```python
from build123d import *

# Parameters (mm, degrees)
F0_R            = 8
F1_DEPTH        = 5
F3_DEPTH        = 5
F3_COPIES_COUNT = 18
F4_R            = 2


# Not quite as in the source:
# - a pattern or mirror of a feature is missing from the dataset's text; its kind, count and spacing are read off the source's solid


with BuildPart() as f1:
    # F0 (on Top) → F1 (new body)
    with BuildSketch(Plane.XY):
        with BuildLine():
            Line((-25, -3), (-10.5830052443, -3))
            ThreePointArc((-10.5830052443, -3), (0, -11), (10.5830052443, -3))
            Line((10.5830052443, -3), (25, -3))
            Line((25, -3), (25, 3))
            Line((25, 3), (10.5830052443, 3))
            ThreePointArc((10.5830052443, 3), (0, 11), (-10.5830052443, 3))
            Line((-10.5830052443, 3), (-25, 3))
            Line((-25, 3), (-25, -3))
        make_face()
        Circle(F0_R, mode=Mode.SUBTRACT)
    extrude(amount=F1_DEPTH)

    # F2 (on Top) → F3 (join)
    with BuildSketch(Plane.XY):
        with BuildLine():
            Line((0, -7.5), (-0.2060079166, -7.9973471063))
            ThreePointArc((-0.2060079166, -7.9973471063), (0, -8), (0.2060079166, -7.9973471063))
            Line((0.2060079166, -7.9973471063), (0, -7.5))
        make_face()
    f3 = extrude(amount=F3_DEPTH)

    # F3_copies: F3 ×18 about axis
    f3_copies_axis = Axis((0, 0, 0), (0, 0, 1))
    for i in range(1, F3_COPIES_COUNT):
        add(f3.rotate(f3_copies_axis, i * 360 / F3_COPIES_COUNT))

    # F4
    f4_edges = [f1.edges().sort_by_distance(p)[0] for p in [
        (-25, 3, 2.5),
        (-25, -3, 2.5),
        (25, 3, 2.5),
        (-10.583005, 3, 2.5),
        (25, -3, 2.5),
        (10.583005, -3, 2.5),
        (-10.583005, -3, 2.5),
        (10.583005, 3, 2.5),
    ]]
    fillet(f4_edges, radius=F4_R)


solid = f1.part
```
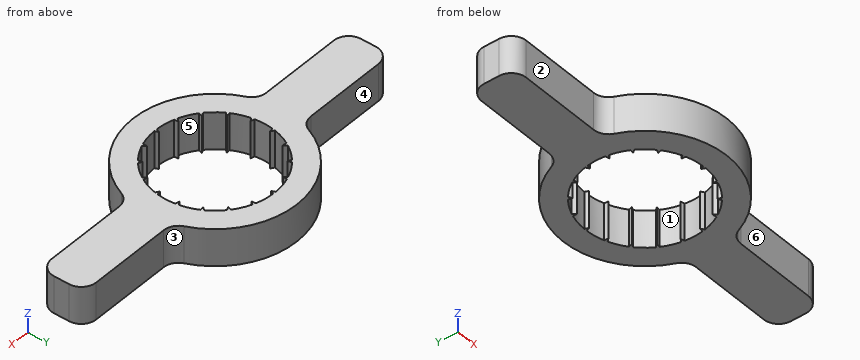
For this review, take the finished solid that the model builds, in its own axes (mm). Face numbers are marked on the shaded views. A direction names the side the tool comes from. Coordinates: 2 decimals unless noted, no trailing zeros. Write each loop counter-clockwise with the first axis right and the second up, starting at its lowest first coordinate (ties: lowest second). Pieces come first, ordered by that corner, then holes.
(1) The part is to be moulded in two halves that separate along Y. For the marked faces 1, 2 and 3, say which applies: +Y half, -Y half, draft (parallel to the pull), parting line (faces both ways), or undercut.
(2) For pin 1 Ø2.5 at (x, z) = (17.5, 3.5) entering from +Y, flat-tipped, find the tip position at first contact; note if it passes through.
(3) Add section A-A on y = 2.5. Give the boundary of the cut face in (x, z).
(4) Wall thickness on probe 1 along X at (y, z) = (5.5, 0.6); probe 2 along Y at (x, z) = (-17, 0.9); probe 3 along X at (y, z) = (-6.75, 3.1): over which ranges is each line inside the solid? List them lowest first.
(5) Add section C-C on y = -9. Give the boundary of the cut face in (x, z).
(6) Add section B-B on x = -13. Give the boundary of the cut face in (y, z).
(7) Tool access review of the marked faces 4, 5 and 6: name each direction out of +Z, -Z, +X, -X, +Y, -Y from which nothing blocks a thin tool from reaching the whole face with its end or side.
Answer sheet:
1. face 1: undercut
1. face 2: -Y half
1. face 3: +Y half
2. pin 1: stops at y = 3
3. outline: (-24.32, 0) - (-7.6, 0) - (-7.6, 5) - (-24.32, 5) - close; (7.6, 0) - (24.32, 0) - (24.32, 5) - (7.6, 5) - close
4. probe 1: x = -9.53 to -5.81, 5.81 to 9.53
4. probe 2: y = -3 to 3
4. probe 3: x = -8.69 to -4.29, 4.29 to 8.69
5. outline: (-6.32, 0) - (6.32, 0) - (6.32, 5) - (-6.32, 5) - close
6. outline: (-3, 0) - (3, 0) - (3, 5) - (-3, 5) - close
7. face 4: +Z, -Z, -X, +Y
7. face 5: +Z, -Z
7. face 6: +Z, -Z, +X, -Y
